Can you work these out from the model? Positions are in its coordinate system, mm. Coordinates: 2 decimals unless noted, no trailing zeros. Order: outer loops, then holes, each group sorted by start corner. A loop starts at its lowest first (then second) coordinate and runs counter-clockwise, first axis right, second up. Notation, with made-up numbers: M 48.5,22 L 56.5,22 A7 ccw 56.5,34 Z; hole C 12.25,46.5 d9. An arc over 180 degrees is marked long. Answer as CSV lines item,"result". Start each with the question number.
1. If we section it at C-C (z = 3.7): Give the number of separate pieces and of enclosed holes in the cut face, plus the area to 3 significant figures.
2. If we mould it in two halves opening along Y, with no side actions, what happens to faces 1 (the face through (123, -132, 5)), 2 (the face through (112.312, -13.45, 2.465))? For each: released by +Y, released by -Y, zero draft, split by the parting line, or undercut.
3. If we section it at B-B (y = -231): List the corners of the cut face in (x, z) for me.
4. Will this pin go through, and if not, where does the flat tip stop? pin 1 (1.5 mm diameter, centred on y = -147, z = 4.5, fed in from -X).
5. If we section it at A-A (y = -84.5): List the corners of the cut face in (x, z) for me, plus the area to 3 significant figures.
6. I need wall thicknesses on line 1 along X through (y, z) = (-59, 0.3); line 2 along Y through (x, z) = (53.5, 1.65); line 3 along Y through (x, z) = (166.46, 3.9) (3 decimals). Which ranges of each line are inside material? Lowest first, please. Write a range as from..to.
```python
from build123d import *

# Parameters (mm, degrees)
SKETCH1_W           = 249.6
SKETCH1_H           = 350.4
SKETCH1_R           = 2.1
SKETCH1_R_2         = 2.5
SKETCH1_R_3         = 1.59
SKETCH1_R_4         = 12.5
SKETCH1_W_2         = 33
SKETCH1_H_2         = 90
BOSS_EXTRUDE1_DEPTH = 5
CUT_EXTRUDE1_DEPTH  = 6
SKETCH12_W          = 249.6
SKETCH12_H          = 5
CUT_EXTRUDE2_DEPTH  = 83


with BuildPart() as part:
    # Sketch1 → Boss-Extrude1 (new body)
    with BuildSketch(Plane.XY):
        with Locations((124.8, -175.2)):
            Rectangle(SKETCH1_W, SKETCH1_H)
        with Locations((104.3, -14)):
            Circle(SKETCH1_R, mode=Mode.SUBTRACT)
        with Locations((245.6, -23.5)):
            Circle(SKETCH1_R_2, mode=Mode.SUBTRACT)
        with Locations((245.6, -74.5)):
            Circle(SKETCH1_R_2, mode=Mode.SUBTRACT)
        with Locations((145.3, -14)):
            Circle(SKETCH1_R, mode=Mode.SUBTRACT)
        with Locations((179.16, -33.375)):
            Circle(SKETCH1_R_3, mode=Mode.SUBTRACT)
        with Locations((179.16, -64.625)):
            Circle(SKETCH1_R_3, mode=Mode.SUBTRACT)
        with Locations((124.8, -14)):
            Circle(SKETCH1_R_4, mode=Mode.SUBTRACT)
        with Locations((141.06, -33.375)):
            Circle(SKETCH1_R_3, mode=Mode.SUBTRACT)
        with Locations((153.76, -33.375)):
            Circle(SKETCH1_R_3, mode=Mode.SUBTRACT)
        with Locations((166.46, -33.375)):
            Circle(SKETCH1_R_3, mode=Mode.SUBTRACT)
        with Locations((141.06, -64.625)):
            Circle(SKETCH1_R_3, mode=Mode.SUBTRACT)
        with Locations((153.76, -64.625)):
            Circle(SKETCH1_R_3, mode=Mode.SUBTRACT)
        with Locations((166.46, -64.625)):
            Circle(SKETCH1_R_3, mode=Mode.SUBTRACT)
        with Locations((83.14, -64.625)):
            Circle(SKETCH1_R_3, mode=Mode.SUBTRACT)
        with Locations((95.84, -64.625)):
            Circle(SKETCH1_R_3, mode=Mode.SUBTRACT)
        with Locations((108.54, -64.625)):
            Circle(SKETCH1_R_3, mode=Mode.SUBTRACT)
        with Locations((83.14, -33.375)):
            Circle(SKETCH1_R_3, mode=Mode.SUBTRACT)
        with Locations((95.84, -33.375)):
            Circle(SKETCH1_R_3, mode=Mode.SUBTRACT)
        with Locations((108.54, -33.375)):
            Circle(SKETCH1_R_3, mode=Mode.SUBTRACT)
        with Locations((70.44, -64.625)):
            Circle(SKETCH1_R_3, mode=Mode.SUBTRACT)
        with Locations((70.44, -33.375)):
            Circle(SKETCH1_R_3, mode=Mode.SUBTRACT)
        with Locations((4, -74.5)):
            Circle(SKETCH1_R_2, mode=Mode.SUBTRACT)
        with Locations((4, -23.5)):
            Circle(SKETCH1_R_2, mode=Mode.SUBTRACT)
        with Locations((201.66, -49)):
            Rectangle(SKETCH1_W_2, SKETCH1_H_2, mode=Mode.SUBTRACT)
        with BuildLine():
            Line((145.8225, -33.375), (145.8225, -38.375))
            ThreePointArc((145.8225, -38.375), (147.41, -39.9625), (148.9975, -38.375))
            Line((148.9975, -38.375), (148.9975, -33.375))
            ThreePointArc((148.9975, -33.375), (147.41, -31.7875), (145.8225, -33.375))
        make_face(mode=Mode.SUBTRACT)
        with BuildLine():
            Line((158.52, -33.375), (158.52, -38.375))
            ThreePointArc((158.52, -38.375), (160.11, -39.965), (161.7, -38.375))
            Line((161.7, -38.375), (161.7, -33.375))
            ThreePointArc((161.7, -33.375), (160.11, -31.785), (158.52, -33.375))
        make_face(mode=Mode.SUBTRACT)
        with BuildLine():
            Line((171.22, -33.375), (171.22, -38.375))
            ThreePointArc((171.22, -38.375), (172.81, -39.965), (174.4, -38.375))
            Line((174.4, -38.375), (174.4, -33.375))
            ThreePointArc((174.4, -33.375), (172.81, -31.785), (171.22, -33.375))
        make_face(mode=Mode.SUBTRACT)
        with BuildLine():
            Line((145.8225, -64.625), (145.8225, -69.625))
            ThreePointArc((145.8225, -69.625), (147.41, -71.2125), (148.9975, -69.625))
            Line((148.9975, -69.625), (148.9975, -64.625))
            ThreePointArc((148.9975, -64.625), (147.41, -63.0375), (145.8225, -64.625))
        make_face(mode=Mode.SUBTRACT)
        with BuildLine():
            Line((158.52, -64.625), (158.52, -69.625))
            ThreePointArc((158.52, -69.625), (160.11, -71.215), (161.7, -69.625))
            Line((161.7, -69.625), (161.7, -64.625))
            ThreePointArc((161.7, -64.625), (160.11, -63.035), (158.52, -64.625))
        make_face(mode=Mode.SUBTRACT)
        with BuildLine():
            Line((171.22, -64.625), (171.22, -69.625))
            ThreePointArc((171.22, -69.625), (172.81, -71.215), (174.4, -69.625))
            Line((174.4, -69.625), (174.4, -64.625))
            ThreePointArc((174.4, -64.625), (172.81, -63.035), (171.22, -64.625))
        make_face(mode=Mode.SUBTRACT)
        with BuildLine():
            Line((103.7775, -33.375), (103.7775, -38.375))
            ThreePointArc((103.7775, -38.375), (102.19, -39.9625), (100.6025, -38.375))
            Line((100.6025, -38.375), (100.6025, -33.375))
            ThreePointArc((100.6025, -33.375), (102.19, -31.7875), (103.7775, -33.375))
        make_face(mode=Mode.SUBTRACT)
        with BuildLine():
            Line((91.08, -33.375), (91.08, -38.375))
            ThreePointArc((91.08, -38.375), (89.49, -39.965), (87.9, -38.375))
            Line((87.9, -38.375), (87.9, -33.375))
            ThreePointArc((87.9, -33.375), (89.49, -31.785), (91.08, -33.375))
        make_face(mode=Mode.SUBTRACT)
        with BuildLine():
            Line((78.38, -33.375), (78.38, -38.375))
            ThreePointArc((78.38, -38.375), (76.79, -39.965), (75.2, -38.375))
            Line((75.2, -38.375), (75.2, -33.375))
            ThreePointArc((75.2, -33.375), (76.79, -31.785), (78.38, -33.375))
        make_face(mode=Mode.SUBTRACT)
        with BuildLine():
            Line((103.7775, -64.625), (103.7775, -69.625))
            ThreePointArc((103.7775, -69.625), (102.19, -71.2125), (100.6025, -69.625))
            Line((100.6025, -69.625), (100.6025, -64.625))
            ThreePointArc((100.6025, -64.625), (102.19, -63.0375), (103.7775, -64.625))
        make_face(mode=Mode.SUBTRACT)
        with BuildLine():
            Line((91.08, -64.625), (91.08, -69.625))
            ThreePointArc((91.08, -69.625), (89.49, -71.215), (87.9, -69.625))
            Line((87.9, -69.625), (87.9, -64.625))
            ThreePointArc((87.9, -64.625), (89.49, -63.035), (91.08, -64.625))
        make_face(mode=Mode.SUBTRACT)
        with BuildLine():
            Line((78.38, -64.625), (78.38, -69.625))
            ThreePointArc((78.38, -69.625), (76.79, -71.215), (75.2, -69.625))
            Line((75.2, -69.625), (75.2, -64.625))
            ThreePointArc((75.2, -64.625), (76.79, -63.035), (78.38, -64.625))
        make_face(mode=Mode.SUBTRACT)
        with Locations((47.94, -49)):
            Rectangle(SKETCH1_W_2, SKETCH1_H_2, mode=Mode.SUBTRACT)
    extrude(amount=BOSS_EXTRUDE1_DEPTH)

    # Sketch11 → Cut-Extrude1 (cut, through all)
    with BuildSketch(Plane.XY.offset(5)):
        with BuildLine():
            Line((66, -220), (0, -220))
            Line((0, -220), (0, -98))
            Line((0, -98), (66, -98))
            ThreePointArc((66, -98), (127, -159), (66, -220))
        make_face()
        with BuildLine():
            Line((234.205987928, -98), (249.6, -98))
            Line((249.6, -98), (249.6, -226.927302483))
            Line((249.6, -226.927302483), (240.532540142, -226.927302483))
            Line((240.532540142, -226.927302483), (240.532540142, -234.598008477))
            Line((240.532540142, -234.598008477), (195.532540142, -234.598008477))
            Line((195.532540142, -234.598008477), (195.532540142, -209.598008477))
            ThreePointArc((195.532540142, -209.598008477), (175.151455799, -140.035097481), (234.205987928, -98))
        make_face()
    extrude(amount=-CUT_EXTRUDE1_DEPTH, mode=Mode.SUBTRACT)

    # Sketch12 → Cut-Extrude2 (cut)
    with BuildSketch(Plane.XZ.offset(350.4)):
        with Locations((124.8, 2.5)):
            Rectangle(SKETCH12_W, SKETCH12_H)
    extrude(amount=-CUT_EXTRUDE2_DEPTH, mode=Mode.SUBTRACT)


solid = part.part
```
Solved:
1,separate pieces,"1"
1,enclosed holes,"37"
1,area,"37,100 mm²"
2,face 1,"zero draft"
2,face 2,"undercut"
3,outline,"M 0,0 L 195.53,0 L 195.53,5 L 0,5 Z; M 240.53,0 L 249.6,0 L 249.6,5 L 240.53,5 Z"
4,pin 1,"x = 125.65"
5,outline,"M 0,0 L 31.44,0 L 31.44,5 L 0,5 Z; M 64.44,0 L 185.16,0 L 185.16,5 L 64.44,5 Z; M 218.16,0 L 249.6,0 L 249.6,5 L 218.16,5 Z"
5,area,"918 mm²"
6,line 1,"0..31.44, 64.44..185.16, 218.16..249.6"
6,line 2,"-267.4..-220, -98..-94, -4..0"
6,line 3,"-267.4..-66.215, -63.035..-34.965, -31.785..0"
